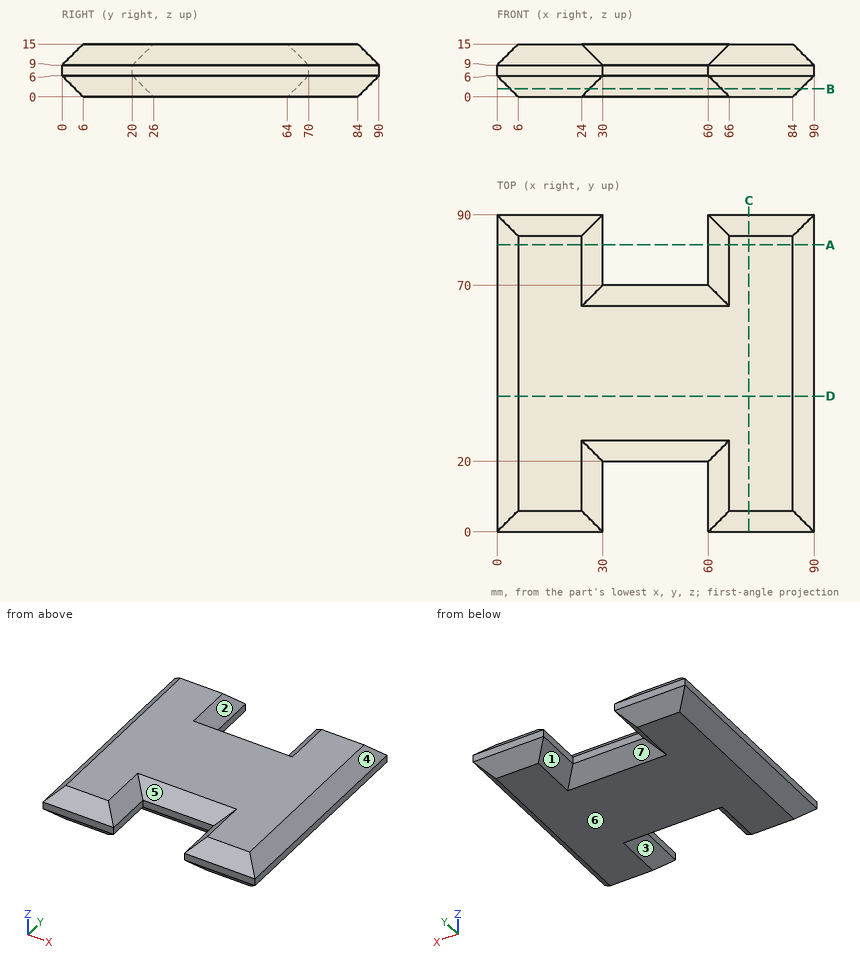
Input: dimensioned drawing with shaded views. Units: mm. Origin: part minimum x, y, z. A direction names the side the tool comes from. Coordinates: 2 decimals unless noted, no trailing zeros. Loops run counter-clockwise (first coordinate to the right, second up) from the corner with the lowest first, then second, coordinate; pieces in that order, holes last. Notation, with made-up numbers: (34, 38.25) -> (48, 38.25) arc R21 ccw to (48, 76.25) -> close; hole circle Ø1 at (-30, 71). An arc over 180 degrees is marked (long way). One line per item, written item: value. Start each with the question number.
Q1. Section query C-C, the plane x = 71.5. Return the cut outline in (y, z), and give its area (3 significant figures).
Q2. Section query A-A, the plane y = 81.5. Return the cut outline in (x, z).
Q3. Contact query for flat-ended pins moving along their axis: P1, Ø3.5, axis at x = 52, z = 8, coming from the +Y side; P2, Ø1.5, axis at x = 40, z = 8, coming from the -Y side; P3, Ø2, axis at y = 75.5, z = 11.5, coming from the +X side. Output: stop coordinate, or through.
Q4. Line query: line 1 along X through (y, z) = (85, 4.5); line 2 along X through (y, z) = (11.5, 3.75); line 3 along Z through (x, y) = (28.5, 20.5). Output: solid intervals per line, ascending.
Q5. Section query B-B, the plane z = 2.25. Return the cut outline in (x, y), and give its area (3 significant figures).
Q6. Mould query, pull axis Z, two halves, no side actions, for the marked faces 1 and 2. Classes: pulls with the +Z half, pulls with the -Z half, needs draft (parallel to the pull), parting line crosses it, or undercut.
Q7. Set-up query: the marked faces 3, 4, 5, 6 and 7. Return all of +Z, -Z, +X, -X, +Y, -Y with unobstructed straight access to the full face (end or side cutting, diameter ignored); none if empty.
Results:
1. outline: (0, 6) -> (6, 0) -> (84, 0) -> (90, 6) -> (90, 9) -> (84, 15) -> (6, 15) -> (0, 9) -> close
1. area: 1,280 mm^2
2. outline: (0, 6) -> (6, 0) -> (24, 0) -> (30, 6) -> (30, 9) -> (24, 15) -> (6, 15) -> (0, 9) -> close; (60, 6) -> (66, 0) -> (84, 0) -> (90, 6) -> (90, 9) -> (84, 15) -> (66, 15) -> (60, 9) -> close
3. P1: y = 70
3. P2: y = 20
3. P3: x = 88.5
4. line 1: 1.5 to 28.5, 61.5 to 88.5
4. line 2: 2.25 to 27.75, 62.25 to 87.75
4. line 3: 4.5 to 10.5
5. outline: (3.75, 3.75) -> (26.25, 3.75) -> (26.25, 23.75) -> (63.75, 23.75) -> (63.75, 3.75) -> (86.25, 3.75) -> (86.25, 86.25) -> (63.75, 86.25) -> (63.75, 66.25) -> (26.25, 66.25) -> (26.25, 86.25) -> (3.75, 86.25) -> close
5. area: 5,310 mm^2
6. face 1: pulls with the -Z half
6. face 2: pulls with the +Z half
7. face 3: -Z, -Y
7. face 4: +Z, +X, +Y, -Y
7. face 5: +Z, -Y
7. face 6: -Z, +X, -X, +Y, -Y
7. face 7: -Z, +Y
